For this review, take the finished solid that the model builds, in its own axes (mm). A direction names the side the tool comes from. Give positions to 0.01 mm unless a question says otherwise; leave off trailing zeros. Write each loop counter-clockwise with the first axis right and the second up, starting at its lowest first coordinate (ties: lowest second). Pieces come first, ordered by that corner, then holes. Notation, with made-up numbers: M 62,60.25 L 119,60.25 A27 ccw 119,93.25 Z; hole C -22.75,88.25 d5. An arc over 180 degrees is marked long. One line per item, written item: value. Start each with the question number.
Item 1: Consider section C-C, the plane x = 5.5. Write out the cut boundary in (y, z).
Item 2: Consider section B-B, the plane y = -2.5. Write out the cut boundary in (x, z), and give its area (3 significant figures).
Item 3: Mouldability with a two-part tool opening along Y and no side actions: class faces 1 (the face through (3.74, -21.08, -41.74)), 2 (the face through (-2.88, -25, -41.6)), 3 (the face through (0, -13, -71.485)) as released by +Y, released by -Y, zero draft, split by the parting line, or undercut.
Item 4: Consider section D-D, the plane x = -6. Write out the cut boundary in (y, z), and give its area (3 significant figures).
Item 5: Tool access review of faces 4 (the face through (2.99, -3.57, -41.71)), 5 (the face through (-5.718, -4.478, -40.722)), 6 (the face through (2.126, -0.885, -41.715)), 7 (the face through (-3.614, -23.027, -40.754)), 8 (the face through (5.718, -20.922, -41.768)): name each direction out of +Z, -Z, +X, -X, +Y, -Y from which nothing blocks a thin tool from reaching the whole face with its end or side.
Item 6: To check wall thickness, follow probe 1 along Z at (x, y) = (4.5, -14); probe 2 along Z at (x, y) = (6.5, -15.75); probe 3 along Y at (x, z) = (-3.5, -20). State the ranges of each line that lie inside material, in increasing order.
Item 7: Clearance check with flat-ended pins moving along their axes: pin 1 Ø2 at (x, z) = (5.5, -52) entering from +Y; pin 2 Ø3 at (y, z) = (-4.5, -62.5) entering from +X. State where each tip first meets the part, or that it passes through.
Item 8: Consider section A-A, the plane z = -51. Write out the cut boundary in (x, y), and give its area (3 significant figures).
```python
from build123d import *

# Parameters (mm, degrees)
F1_DEPTH = 25.4
F2_SIZE  = 5.08
F3_R     = 5.08
F4_DEPTH = 2.54
F5_DEPTH = 2.54
F6_DEPTH = 2.54
F7_DEPTH = 2.54


with BuildPart() as f1:
    # F0 (on Front) → F1 (new body)
    with BuildSketch(Plane.XZ):
        Polygon((-8.0913305283, -71.4852660894), (8.0913305283, -71.4852660894), (8.0913305283, -11.2523705258), (-8.0913305283, -10.7631014283), align=None)
    extrude(amount=F1_DEPTH)

    # F2
    f2_edges = [f1.edges().sort_by_distance(p)[0] for p in [
        (8.091331, -25.4, -41.368818),
        (-8.091331, -25.4, -41.124184),
        (-8.091331, 0, -41.124184),
        (8.091331, 0, -41.368818),
    ]]
    chamfer(f2_edges, length=F2_SIZE)

    # F3
    f3_edges = [f1.edges().sort_by_distance(p)[0] for p in [
        (-3.011331, 0, -41.200979),
        (-8.091331, -20.32, -41.124184),
        (-8.091331, -5.08, -41.124184),
        (8.091331, -5.08, -41.368818),
        (8.091331, -20.32, -41.368818),
        (-3.011331, -25.4, -41.200979),
        (3.011331, -25.4, -41.292024),
    ]]
    fillet(f3_edges, radius=F3_R)

    # F4 (cut): a face of the model
    f4_faces = [f1.faces().sort_by_distance(p)[0] for p in [
        (-5.5515144762, -22.859816052, -41.1625783561),
    ]]
    extrude(f4_faces, amount=-F4_DEPTH, mode=Mode.SUBTRACT)

    # F5 (cut): a face of the model
    f5_faces = [f1.faces().sort_by_distance(p)[0] for p in [
        (-5.5515144762, -2.540183948, -41.1625783561),
    ]]
    extrude(f5_faces, amount=-F5_DEPTH, mode=Mode.SUBTRACT)

    # F6 (cut): a face of the model
    f6_faces = [f1.faces().sort_by_distance(p)[0] for p in [
        (4.8068429061, -1.7955123778, -41.3191664522),
    ]]
    extrude(f6_faces, amount=-F6_DEPTH, mode=Mode.SUBTRACT)

    # F7 (cut): a face of the model
    f7_faces = [f1.faces().sort_by_distance(p)[0] for p in [
        (5.5511455564, -22.8601849718, -41.3304181334),
    ]]
    extrude(f7_faces, amount=-F7_DEPTH, mode=Mode.SUBTRACT)


solid = f1.part
```
Model answer:
1. outline: M -22.91,-11.17 L -20.7,-11.21 L -20.7,-71.49 L -4.7,-71.49 L -4.7,-11.21 L -2.49,-11.17 Z
2. outline: M -3.49,-71.49 L 1.92,-71.49 L 1.92,-11.12 L 5.51,-11.17 L -3.49,-10.9 Z
2. area: 327 mm2
3. face 1: undercut
3. face 2: released by -Y
3. face 3: zero draft
4. outline: M -21.2,-71.49 L -4.2,-71.49 L -4.2,-10.83 L -21.2,-10.83 Z
4. area: 1,030 mm2
5. face 4: -Z
5. face 5: +Z, -Z, +Y
5. face 6: -Z, +X
5. face 7: +Z, -Z, -X
5. face 8: -Z, -Y
6. probe 1: z = -71.49 to -11.14
6. probe 2: z = -71.49 to -11.2
6. probe 3: y = -24.69 to -22.91, -21.32 to -4.08, -2.49 to -0.71
7. pin 1: stops at y = -3.7
7. pin 2: stops at x = 7.95
8. outline: M -8.09,-18.22 A5.08 ccw -6.6,-21.81 L -4.81,-20.01 L -2.7,-22.12 L -4.5,-23.91 A5.08 ccw -0.91,-25.4 L 0.91,-25.4 A5.08 ccw 4.5,-23.91 L 2.7,-22.12 L 4.81,-20.01 L 6.6,-21.81 A5.08 ccw 8.09,-18.22 L 8.09,-7.18 A5.08 ccw 6.6,-3.59 L 4.81,-5.39 L 1.22,-1.8 L 3.01,0 L -0.91,0 A5.08 ccw -4.5,-1.49 L -2.7,-3.28 L -4.81,-5.39 L -6.6,-3.59 A5.08 ccw -8.09,-7.18 Z
8. area: 320 mm2
